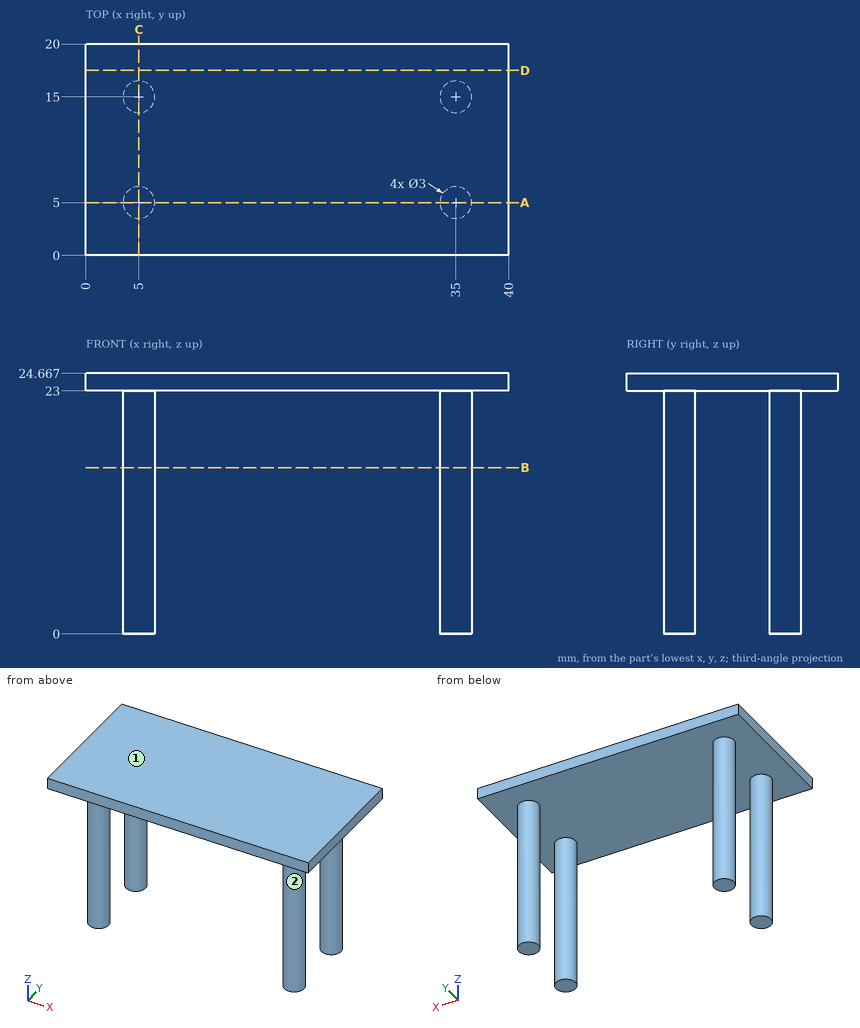
Here's the drawing with two shaded views (mm, measured from the low corner). I have some questions. Give positions to 0.01 mm unless a question says otherwise; leave off trailing zeros. Loops run counter-clockwise (first coordinate to the right, second up) from the corner with the lowest first, then second, coordinate; pieces in that order, holes last. Notation, with made-up numbers: (71.25, -21.75) -> (76.25, -21.75) arc R31 cw to (76.25, 5.25) -> close; hole circle Ø10 at (22, 49). An arc over 180 degrees is marked (long way). One line per item, written item: value.
Q1. Suppose I cut it at B-B on z = 15.75. Please give me the cut outline in (x, y).
Answers follow:
outline: circle Ø3 at (5, 5); circle Ø3 at (5, 15); circle Ø3 at (35, 5); circle Ø3 at (35, 15)
Q2. We'd pull the mould along X, two halves only. Please class the marked faces 1 and 2: pulls with the +X half, pulls with the -X half, needs draft (parallel to the pull), parting line crosses it, or undercut.
Answers follow:
face 1: needs draft
face 2: undercut
Q3. Suppose I cut it at D-D on y = 17.5. Please give me the cut outline in (x, z).
Answers follow:
outline: (0, 23) -> (40, 23) -> (40, 24.67) -> (0, 24.67) -> close
Q4. Suppose I cut it at C-C on x = 5. Please give me the cut outline in (y, z), then the cut area to 3 significant figures.
Answers follow:
outline: (0, 23) -> (3.5, 23) -> (3.5, 0) -> (6.5, 0) -> (6.5, 23) -> (13.5, 23) -> (13.5, 0) -> (16.5, 0) -> (16.5, 23) -> (20, 23) -> (20, 24.67) -> (0, 24.67) -> close
area: 171 mm^2
Q5. Suppose I cut it at A-A on y = 5. Please give me the cut outline in (x, z).
Answers follow:
outline: (0, 23) -> (3.5, 23) -> (3.5, 0) -> (6.5, 0) -> (6.5, 23) -> (33.5, 23) -> (33.5, 0) -> (36.5, 0) -> (36.5, 23) -> (40, 23) -> (40, 24.67) -> (0, 24.67) -> close
Q6. If I drill on line 1 along Z through (x, y) = (19.5, 2.75); line 2 along X through (y, z) = (5.75, 5); line 3 along X through (y, z) = (16, 6), over which ranges is the centre line in solid material (lowest first)?
Answers follow:
line 1: 23 to 24.67
line 2: 3.7 to 6.3, 33.7 to 36.3
line 3: 3.88 to 6.12, 33.88 to 36.12
Q7. I'm going to push flat-ended pins straight in: pin 1 Ø6 at (x, z) = (8, 13.5) entering from +Y; pin 2 Ø5 at (x, y) = (32, 12) entering from -Z; pin 3 Ø1.5 at (x, z) = (6.5, 15.5) entering from +Y. Where does each tip first touch, or does it pass through?
Answers follow:
pin 1: y = 16.5
pin 2: z = 23
pin 3: y = 16.3
